Source: CAD feature listing. Evaluate the final solid. Frame: model axes, mm. A direction names the side the tool comes from. Give positions to 0.01 mm unless a question says otherwise; leave off trailing zeros. Loops run counter-clockwise (first coordinate to the right, second up) from the corner with the lowest first, then second, coordinate; pieces in that order, holes last. Notation, with made-up numbers: M 49.5,17 L 91.5,17 A23 cw 91.5,49 Z; hole C 27,25.25 d8. An arc over 180 degrees is marked long. Answer in a Markdown table with one row per item.
```python
from build123d import *

# Parameters (mm, degrees)
SKETCH1_W           = 110
SKETCH1_H           = 28
BOSS_EXTRUDE1_DEPTH = 5
SKETCH2_W           = 110
SKETCH2_H           = 32
BOSS_EXTRUDE2_DEPTH = 6.78
SKETCH3_R           = 1.5
CUT_EXTRUDE1_DEPTH  = 117.674761624
SKETCH4_R           = 1.5
CUT_EXTRUDE2_DEPTH  = 117.508748169
FILLET1_R           = 5
SKETCH5_W           = 6
SKETCH5_H           = 3
BOSS_EXTRUDE3_DEPTH = 6
SKETCH6_R           = 1.5
CUT_EXTRUDE3_DEPTH  = 6


with BuildPart() as part:
    # Sketch1 → Boss-Extrude1 (new body)
    with BuildSketch(Plane(origin=(0, 0, 0), x_dir=(1, 0, 0), z_dir=(0, 1, 0))):
        with Locations((55, 14)):
            Rectangle(SKETCH1_W, SKETCH1_H)
    extrude(amount=BOSS_EXTRUDE1_DEPTH)

    # Sketch2 → Boss-Extrude2 (add)
    with BuildSketch(Plane(origin=(0, 0, -28), x_dir=(-1, 0, 0), z_dir=(0, 0, -1))):
        with Locations((-55, 16)):
            Rectangle(SKETCH2_W, SKETCH2_H)
    extrude(amount=-BOSS_EXTRUDE2_DEPTH)

    # Sketch3 → Cut-Extrude1 (cut, through all)
    with BuildSketch(Plane(origin=(0, 5, 0), x_dir=(-1, 0, 0), z_dir=(0, 1, 0))):
        with Locations(Location((-13.16, -17.28, 0), (0, 0, 90))):
            Circle(SKETCH3_R)
        with Locations(Location((-53.16, -17.28, 0), (0, 0, 90))):
            Circle(SKETCH3_R)
        with Locations(Location((-93.16, -17.28, 0), (0, 0, 90))):
            Circle(SKETCH3_R)
    extrude(amount=-CUT_EXTRUDE1_DEPTH, mode=Mode.SUBTRACT)

    # Sketch4 → Cut-Extrude2 (cut, through all)
    with BuildSketch(Plane.XY.offset(-21.22)):
        with Locations((45, 8.5)):
            Circle(SKETCH4_R)
        with Locations((65, 8.5)):
            Circle(SKETCH4_R)
        with Locations((45, 28.5)):
            Circle(SKETCH4_R)
        with Locations((65, 28.5)):
            Circle(SKETCH4_R)
    extrude(amount=-CUT_EXTRUDE2_DEPTH, mode=Mode.SUBTRACT)

    # Fillet1
    fillet1_edges = [part.edges().sort_by_distance(p)[0] for p in [
        (0, 16, -28),
        (110, 16, -28),
    ]]
    fillet(fillet1_edges, radius=FILLET1_R)

    # Sketch5 → Boss-Extrude3 (add)
    with BuildSketch(Plane(origin=(0, 5, 0), x_dir=(-1, 0, 0), z_dir=(0, 1, 0))):
        with Locations((-33, -1.5)):
            Rectangle(SKETCH5_W, SKETCH5_H)
        with Locations((-77, -1.5)):
            Rectangle(SKETCH5_W, SKETCH5_H)
    extrude(amount=BOSS_EXTRUDE3_DEPTH)

    # Sketch6 → Cut-Extrude3 (cut)
    with BuildSketch(Plane.XY):
        with Locations((33, 8)):
            Circle(SKETCH6_R)
        with Locations((77, 8)):
            Circle(SKETCH6_R)
    extrude(amount=-CUT_EXTRUDE3_DEPTH, mode=Mode.SUBTRACT)


solid = part.part
```
Q1. Mould query, pull axis Y, two halves, no side actions, for faces 1 (the flat face through (33, 11, -1)), 2 (the cylindrical face through (78.386, 7.425, -1.479)), 3 (the cylindrical face through (31.5, 8.07, -1.48)), 4 (the flat face through (110, 4, -15)). Classes: +Y half, -Y half, draft (parallel to the pull), parting line (faces both ways), or undercut.
Values follow:
| item | result |
|---|---|
| face 1 | +Y half |
| face 2 | undercut |
| face 3 | undercut |
| face 4 | draft |
Q2. Contact query for flat-ended pins moving along their axis: pin 1 Ø8 at (x, y) = (42.5, 10.5) entering from +Z; pin 2 Ø2.5 at (x, z) = (33.5, -1.5) entering from +Y; pin 3 Ø2.5 at (y, z) = (8, -2) entering from +X. Output: stop coordinate, or through.
Values follow:
| item | result |
|---|---|
| pin 1 | z = -21.22 |
| pin 2 | y = 11 |
| pin 3 | x = 80 |
Q3. Ray query, probe 1 along X at (y, z) = (1.1, -17.28); probe 2 along Y at (x, z) = (45, -26.25); probe 3 along Y at (x, z) = (33, -0.8). Return the intervals inside material, ascending. Write a range as from..to.
Values follow:
| item | result |
|---|---|
| probe 1 | 0..11.66, 14.66..51.66, 54.66..91.66, 94.66..110 |
| probe 2 | 0..7, 10..27, 30..32 |
| probe 3 | 0..6.5, 9.5..11 |
Q4. Section query A-A (x = 65). Output: boundary loops of the cut face in (y, z), plus the area to 3 significant figures.
Values follow:
| item | result |
|---|---|
| outline | M 0,-28 L 7,-28 L 7,-21.22 L 5,-21.22 L 5,0 L 0,0 Z; M 10,-28 L 27,-28 L 27,-21.22 L 10,-21.22 Z; M 30,-28 L 32,-28 L 32,-21.22 L 30,-21.22 Z |
| area | 282 mm^2 |
Q5. Section query C-C (z = -17.28). Output: boundary loops of the cut face in (x, y), plus the area to 3 significant figures.
Values follow:
| item | result |
|---|---|
| outline | M 0,0 L 11.66,0 L 11.66,5 L 0,5 Z; M 14.66,0 L 51.66,0 L 51.66,5 L 14.66,5 Z; M 54.66,0 L 91.66,0 L 91.66,5 L 54.66,5 Z; M 94.66,0 L 110,0 L 110,5 L 94.66,5 Z |
| area | 505 mm^2 |
Q6. Reachability of faces 5 (the flat face through (77, 11, -1)), 6 (the flat face through (54, 3, 0)), 7 (the flat face through (80, 8, -2)), 8 (the flat face through (78.4, 6.6, -3)) from +Z, -Z, +X, -X, +Y, -Y: full face, straight path, thin tool, end or side. Return the list, or none.
Values follow:
| item | result |
|---|---|
| face 5 | +Z, +X, -X, +Y |
| face 6 | +Z, +X, -X, +Y, -Y |
| face 7 | +Z, +X, +Y |
| face 8 | +X, -X, +Y |
Q7. Section query B-B (x = 77). Output: boundary loops of the cut face in (y, z).
Values follow:
| item | result |
|---|---|
| outline | M 0,-28 L 32,-28 L 32,-21.22 L 5,-21.22 L 5,-3 L 6.5,-3 L 6.5,0 L 0,0 Z; M 9.5,-3 L 11,-3 L 11,0 L 9.5,0 Z |
Q8. Section query D-D (y = 24). Output: boundary loops of the cut face in (x, z).
Values follow:
| item | result |
|---|---|
| outline | M 0,-23 A5 ccw 5,-28 L 105,-28 A5 ccw 110,-23 L 110,-21.22 L 0,-21.22 Z |
